Can you work these out from the model? Positions are in its coordinate system, mm. Face numbers are marked on the shaded views. A direction names the side the tool comes from. Round coordinates to 2 decimals unless told otherwise and drop trailing zeros. Order: outer loops, then holes, each group sorted by start corner. A loop starts at its lowest first (then second) coordinate and runs counter-clockwise, first axis right, second up. Notation, with made-up numbers: (-10.5, -12.75) -> (34.5, -12.75) arc R9 ccw to (34.5, -1.75) -> close; hole circle Ø8 at (20, 10.25). An arc over 180 degrees is marked (long way). One line per item, written item: value.
Autodesk Inventor part; units mm, degrees
ref_plane "YZ Plane" through (0, 0, 0) normal (1, 0, 0) x (0, 1, 0)
ref_plane "XZ Plane" through (0, 0, 0) normal (0, 1, 0) x (-1, 0, 0)
ref_plane "XY Plane" through (0, 0, 0) normal (0, 0, 1) x (1, 0, 0)
sketch "Sketch1" plane through (0, 0, 0) normal (0, 0, 1) x (1, 0, 0)
  circle A0 centre (0, 0) radius 29.5
  circle A1 centre (20, 0) radius 3.375
  circle A2 centre (-20, 0) radius 3.375
  line L0 (0, -27.5) -> (-4.0078, -26.1952)
  line L1 (0, -27.5) -> (4.0078, -26.1952)
  arc A3 (-24.1091, -11) -> (-4.0078, -26.1952) centre (0, 0) ccw
  arc A4 (4.0078, -26.1952) -> (24.1091, -11) centre (0, 0) ccw
  line L2 (4.0076, 26.1952) -> (0, 27.5)
  line L3 (0, 27.5) -> (-4.0076, 26.1952)
  arc A5 (24.1091, 11) -> (4.0076, 26.1952) centre (0, 0) ccw
  arc A6 (-4.0076, 26.1952) -> (-24.1091, 11) centre (0, 0) ccw
  arc A7 (20.1829, 7.4978) -> (20.1829, -7.4978) centre (20, 0) ccw
  arc A8 (-20.1829, -7.4978) -> (-20.1829, 7.4978) centre (-20, 0) ccw
  arc A9 (-20, -7.5) -> (-24.1091, -11) centre (-20.1402, -11.4975) ccw
  arc A10 (-24.1091, 11) -> (-20, 7.5) centre (-20.1402, 11.4975) ccw
  arc A11 (24.1091, -11) -> (20, -7.5) centre (20.1402, -11.4975) ccw
  arc A12 (20, 7.5) -> (24.1091, 11) centre (20.1402, 11.4975) ccw
  dimension "d46" = 59
  dimension "d49" = 6.75
  dimension "d50" = 6.75
  dimension "d105" = 4
  dimension "d106" = 4
  dimension "d107" = 4
  dimension "d109" = 4
extrude "Extrusion1" add sketch "Sketch1" along normal blind 35
sketch "Sketch9" plane through (0, 0, 0) normal (0, 0, -1) x (-1, 0, 0)
  circle A0 centre (-20, 0) radius 3.375
  circle A1 centre (20, 0) radius 3.375
  line L0 (20, -6.5) -> (25.6292, -3.25)
  line L1 (25.6292, -3.25) -> (25.6292, 3.25)
  line L2 (25.6292, 3.25) -> (20, 6.5)
  line L3 (20, 6.5) -> (14.3708, 3.25)
  line L4 (14.3708, 3.25) -> (14.3708, -3.25)
  line L5 (14.3708, -3.25) -> (20, -6.5)
  line L6 (-20, -6.5) -> (-14.3708, -3.25)
  line L7 (-14.3708, -3.25) -> (-14.3708, 3.25)
  line L8 (-14.3708, 3.25) -> (-20, 6.5)
  line L9 (-20, 6.5) -> (-25.6292, 3.25)
  line L10 (-25.6292, 3.25) -> (-25.6292, -3.25)
  line L11 (-25.6292, -3.25) -> (-20, -6.5)
  point P0 (0, 0)
  point P1 (0, 0)
extrude "Extrusion11" cut sketch "Sketch9" against normal blind 3
extrude "Extrusion12" add sketch "Sketch1" against normal blind 3 contours A0 | L0 A3 A9 A8 A10 A6 L3 L2 A5 A12 A7 A11 A4 L1
extrude "Extrusion13" cut sketch "Sketch9" along normal blind 3
sketch "Sketch10" plane through (0, 0, 35) normal (0, 0, 1) x (1, 0, 0)
  arc A0 (-24.1091, -11) -> (-4.0078, -26.1952) centre (0, 0) ccw
  line L0 (0, -26.5) -> (12.9615, -26.5)
  line L1 (27.1662, -11.5) -> (23.8747, -11.5)
  arc A1 (24.1091, 11) -> (4.0076, 26.1952) centre (0, 0) ccw
  line L2 (0, 26.5) -> (-12.9615, 26.5)
  line L3 (-27.1662, 11.5) -> (-23.8747, 11.5)
  arc A2 (12.9615, -26.5) -> (27.1662, -11.5) centre (0, 0) ccw
  arc A3 (-12.9615, 26.5) -> (-27.1662, 11.5) centre (0, 0) ccw
  arc A4 (0, -26.5) -> (23.8747, -11.5) centre (0, 0) ccw
  arc A5 (0, 26.5) -> (-23.8747, 11.5) centre (0, 0) ccw
  point P0 (24.1091, -11)
  point P1 (-24.1091, 11)
extrude "Extrusion14" cut sketch "Sketch10" against normal blind 25
sketch "Sketch11" plane through (0, 0, 35) normal (0, 0, 1) x (1, 0, 0)
  line L0 (12.9615, -26.5) -> (3.0715, -26.5)
  line L1 (12.9615, -26.5) -> (22.9615, -26.5)
  line L2 (22.9615, -26.5) -> (22.9615, -29.5)
  arc A0 (-27.1662, 11.5) -> (12.9615, -26.5) centre (0, 0) ccw
  line L3 (0, -29.5) -> (22.9615, -29.5)
  line L4 (12.9615, -26.5) -> (3.0715, -26.5)
  line L5 (3.0715, -26.5) -> (0, -27.5)
  line L6 (0, -27.5) -> (0, -29.5)
  circle A1 centre (0, 0) radius 29.5
  line L7 (-12.9667, 26.4974) -> (-22.9667, 26.4974)
  line L8 (-22.9667, 26.4974) -> (-22.9667, 29.7944)
  line L9 (0, 29.5) -> (-22.9667, 29.7944)
  line L10 (-12.9667, 26.4974) -> (-3.0793, 26.4974)
  line L11 (0, 27.5) -> (-4.0076, 26.1952)
  line L12 (0, 27.5) -> (0, 29.5)
  dimension "d93" = 10
  dimension "d94" = 10
extrude "Extrusion15" add sketch "Sketch11" against normal blind 38 contours A0 L6 L5 L0 | L1 L2 L3 A0 | A1 L7 L8 L9
properties part number "BatteryIsolator"
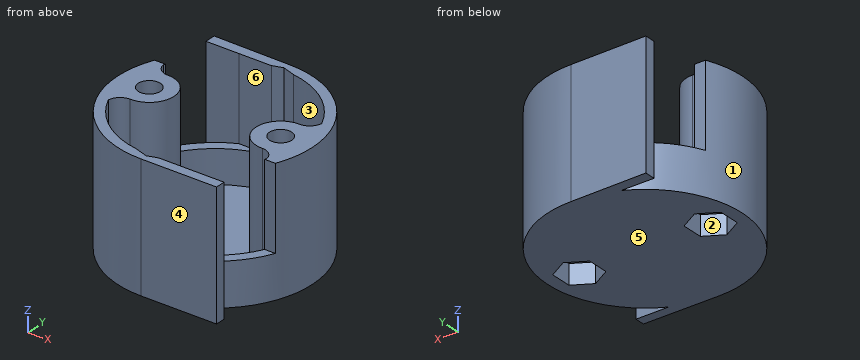
Q1. I want a section at B-B on z = 17.5. Give the number of separate pieces and of enclosed holes in the cut face, plus the area to 3 significant figures.
Answers below:
separate pieces: 2
enclosed holes: 2
area: 782 mm^2
Q2. On a 3-axis mill with a long thin cutter (end or side, diameter ignored), from which of +Z, -Z, +X, -X, +Y, -Y can I reach the whole of each face in a straight line? I mean the marked faces 1, 2 and 3. Say none if no direction works.
Answers below:
face 1: +Z, -Z, -X
face 2: -Z
face 3: +Z
Q3. I want a section at A-A on y = 0. List the corners of the cut face in (x, z) for me (3 decimals), plus the area to 3 significant figures.
Answers below:
outline: (-29.5, -3) -> (-25.629, -3) -> (-25.629, 3) -> (-23.375, 3) -> (-23.375, 35) -> (-29.5, 35) -> close; (-16.625, 3) -> (-14.371, 3) -> (-14.371, -3) -> (14.371, -3) -> (14.371, 3) -> (16.625, 3) -> (16.625, 35) -> (12.5, 35) -> (12.5, 0) -> (-12.5, 0) -> (-12.5, 35) -> (-16.625, 35) -> close; (23.375, 3) -> (25.629, 3) -> (25.629, -3) -> (29.5, -3) -> (29.5, 35) -> (23.375, 35) -> close
area: 800 mm^2
Q4. Will these pins go through, and if not, where does the flat tip stop? pin 1 Ø6 at (x, z) = (16, 20.5) entering from +Y; pin 2 Ø6 at (y, z) = (-6.5, 30.5) entering from +X; pin 3 Ø16.5 at (x, y) = (17, -15.5) entering from +Z; pin 4 Ø8 at (x, z) = (19.5, 24.5) entering from +Y.
Answers below:
pin 1: y = 26.48
pin 2: x = 29.29
pin 3: z = 35
pin 4: y = 25.1
Q5. I want a section at D-D on y = 24. List the corners of the cut face in (x, z) for me, plus the area to 3 significant figures.
Answers below:
outline: (-17.15, -3) -> (17.15, -3) -> (17.15, 35) -> (11.24, 35) -> (11.24, 0) -> (-11.24, 0) -> (-11.24, 10) -> (-17.15, 10) -> close
area: 369 mm^2
Q6. We'd pull the mould along Y, two halves only. Please class the marked faces 4, 5 and 6: released by +Y, released by -Y, zero draft, split by the parting line, or undercut.
Answers below:
face 4: released by -Y
face 5: zero draft
face 6: undercut
Q7. I want a section at C-C on y = -21. List the corners of the cut face in (x, z) for me.
Answers below:
outline: (-20.72, -3) -> (20.72, -3) -> (20.72, 10) -> (16.16, 10) -> (16.16, 0) -> (-16.16, 0) -> (-16.16, 35) -> (-20.72, 35) -> close
Q8. Please list where these lines run through material, in increasing order: line 1 along X through (y, z) = (0, 21.5) (3 decimals); line 2 along Y through (x, z) = (-20, 24.5) (3 decimals); line 3 along Y through (x, z) = (20, 12.5) (3 decimals).
Answers below:
line 1: -29.5 to -23.375, -16.625 to -12.5, 12.5 to 16.625, 23.375 to 29.5
line 2: -21.685 to -17.385, -7.5 to -3.375, 3.375 to 7.5, 26.497 to 29.756
line 3: -29.5 to -26.5, -7.5 to -3.375, 3.375 to 7.5, 17.385 to 21.685
